The model under review builds one solid part; all positions refer to its coordinate system, in mm. A direction names the side the tool comes from. Give positions to 0.01 mm unless a question says otherwise; leave off trailing zeros. Loops run counter-clockwise (first coordinate to the right, second up) from the corner with the lowest first, then second, coordinate; pieces in that order, holes last. Notation, with made-up numbers: M -34.75,-1.75 L -22.75,-1.75 A10 cw -22.75,13.25 Z; hole C 52.5,46 d5. An arc over 180 degrees is marked long. Return JSON: item names as keys, results as strings.
Autodesk Inventor part; units mm, degrees
ref_plane "YZ Plane" through (0, 0, 0) normal (1, 0, 0) x (0, 1, 0)
ref_plane "XZ Plane" through (0, 0, 0) normal (0, 1, 0) x (-1, 0, 0)
ref_plane "XY Plane" through (0, 0, 0) normal (0, 0, 1) x (1, 0, 0)
sketch "Boceto1" plane through (0, 0, 0) normal (1, 0, 0) x (0, 1, 0)
  line L0 (0, 8) -> (10, 8)
  line L1 (10, 8) -> (10, 20)
  line L2 (10, 20) -> (0, 20)
  line L3 (20, 60) -> (0, 40)
  line L4 (0, 0) -> (20, 0)
  line L5 (40, 20) -> (20, 0)
  line L6 (20, 60) -> (40, 60)
  line L7 (0, 20) -> (0, 40)
  line L8 (0, 8) -> (0, 0)
  line L9 (40, 60) -> (120, 60)
  line L10 (120, 60) -> (120, 20)
  line L11 (80, 20) -> (80, 0)
  line L12 (80, 0) -> (120, 0)
  line L13 (120, 0) -> (120, 20)
  line L14 (40, 20) -> (80, 20)
  line L15 (120, 60) -> (115, 60)
  line L16 (120, 55) -> (120, 60)
  line L17 (20, 60) -> (25, 60)
  line L18 (120, 0) -> (115, 0)
  line L19 (120, 5) -> (120, 0)
  line L20 (0, 35) -> (0, 40)
  line L21 (0, 0) -> (5, 0)
  line L22 (0, 5) -> (0, 0)
  circle A0 centre (115, 55) radius 1.5
  circle A1 centre (115, 5) radius 1.5
  circle A2 centre (25, 55) radius 1.5
  circle A3 centre (5, 35) radius 1.5
  circle A4 centre (5, 5) radius 1.5
  line L23 (80, 0) -> (85, 0)
  line L24 (80, 5) -> (80, 0)
  circle A5 centre (85, 5) radius 1.5
  dimension "d2" = 8
  dimension "d3" = 10
  dimension "d4" = 12
  dimension "d5" = 40
  dimension "d7" = 20
  dimension "d11" = 20
  dimension "d12" = 20
  dimension "d13" = 20
  dimension "d16" = 100
  dimension "d17" = 60
  dimension "d18" = 40
  dimension "d27" = 3
  dimension "d28" = 3
  dimension "d29" = 3
  dimension "d30" = 3
  dimension "d31" = 3
  dimension "d34" = 3
  dimension "d35" = 5
  dimension "d36" = 5
  dimension "d37" = 5
  dimension "d38" = 5
  dimension "d39" = 5
  dimension "d40" = 5
  dimension "d41" = 5
  dimension "d42" = 5
  dimension "d43" = 5
  dimension "d44" = 5
  dimension "d45" = 5
  dimension "d46" = 5
extrude "Extrusión1" add sketch "Boceto1" along normal blind 5
sketch "Boceto2" plane through (5, 0, 0) normal (1, 0, 0) x (0, 0, -1)
  point P0 (0, 0)
sketch "Boceto3" plane through (5, 0, 0) normal (1, 0, 0) x (0, 0, -1)
  circle A0 centre (-25, 45) radius 1.5
  line L0 (-20, 40) -> (-20, 80)
  circle A1 centre (-45, 45) radius 1.5
  point P0 (0, 0)
  dimension "d49" = 3
  dimension "d50" = 5
  dimension "d51" = 5
  dimension "d52" = 3
  dimension "d53" = 20
  dimension "d54" = 5
extrude "Extrusión2" cut sketch "Boceto3" against normal blind 5
sketch "Boceto4" plane through (0, 0, 20) normal (0, -1, 0) x (1, 0, 0)
  point P0 (0, -20)
sketch "Boceto5" plane through (0, 0, 0) normal (0, -1, 0) x (1, 0, 0)
  circle A0 centre (2.5, 2.5) radius 1.5
  line L0 (0, 0) -> (5, 0)
  line L1 (0, 8) -> (0, 0)
  dimension "d57" = 3
  dimension "d58" = 2.5
  dimension "d59" = 2.5
extrude "Extrusión3" cut sketch "Boceto5" against normal blind 3
sketch "Boceto6" plane through (5, 0, 0) normal (1, 0, 0) x (0, 0, -1)
  line L0 (-8, 0) -> (0, 0)
  line L1 (-20.5, 10.5) -> (-7.5, 10.5)
  line L2 (-7.5, 10.5) -> (-7.5, 0)
  line L3 (-7.5, 0) -> (-20.5, 0)
  line L4 (-20.5, 0) -> (-20.5, 10.5)
  line L5 (-8, 10) -> (-8, 0)
  line L6 (-20, 0) -> (-20, 10)
  line L7 (-20, 10) -> (-8, 10)
  point P0 (-20.5, 5.25)
  dimension "d62" = 0.5
  dimension "d63" = 0.5
  dimension "d64" = 0.5
extrude "Extrusión4" cut sketch "Boceto6" against normal blind 10
sketch "Boceto7" plane through (5, 0, 0) normal (1, 0, 0) x (0, 0, -1)
  point P0 (0, 0)
sketch "Boceto8" plane through (0, 0, 40) normal (0, -1, 0) x (1, 0, 0)
  line L0 (5, -3.5) -> (0, -3.5)
  circle A0 centre (2.5, -3.5) radius 1.5
  point P0 (0, -40)
  dimension "d67" = 3
extrude "Extrusión5" cut sketch "Boceto8" against normal blind 3
sketch "Boceto9" plane through (5, 0, 0) normal (1, 0, 0) x (0, 0, -1)
  circle A0 centre (-35, 5) radius 1.5
  circle A1 centre (-35, 5) radius 1.5
  circle A2 centre (-5, 5) radius 1.5
  circle A3 centre (-5, 5) radius 1.5
  point P0 (0, 0)
extrude "Extrusión6" add sketch "Boceto9" against normal blind 5
properties part number "Lateral"
1) The part is to be moulded in two halves that separate along X. For faces 5 (the face through (0, 59, 37)), 6 (the face through (2, 3, 3)), 7 (the face through (2.46, 23.5, 54.93)), 8 (the face through (5, 59, 37)), say which applies: released by +X, released by -X, zero draft, split by the parting line, or undercut.
From the geometry:
{"face 5": "released by -X", "face 6": "undercut", "face 7": "zero draft", "face 8": "released by +X"}
2) Consider section A-A on y = 25. Write out the cut boundary in (x, z).
From the geometry:
{"outline": "M 0,5 L 5,5 L 5,53.5 L 0,53.5 Z; M 0,56.5 L 5,56.5 L 5,60 L 0,60 Z"}
3) Wall thickness on L1, parallel to Y at x = 3.75, z = 25; L2, parallel to Y at x = 4.8, z = 56; L3, parallel to Y at x = 2.25, z = 45: over which ranges is each line inside the solid? List them lowest first. Write a range as from..to.
From the geometry:
{"L1": "0..43.5, 46.5..120", "L2": "16..23.88, 26.12..113.88, 116.12..120", "L3": "5..43.5, 46.5..120"}
4) Insertion check: pin 1 (1 mm diameter, centred on x = 3, z = 23, fed in from -Y); pin 2 (1.8 mm diameter, centred on y = 45, z = 45, fed in from -X); pin 3 (1.5 mm diameter, centred on x = 3.5, y = 6, fed in from +Z); pin 4 (1.5 mm diameter, centred on x = 2.5, y = 54, fed in from -Z). Each pin has a flat end and moves straight along its axis. Give the tip position at first contact, or say it passes through.
From the geometry:
{"pin 1": "y = 0", "pin 2": "through", "pin 3": "z = 46.75", "pin 4": "z = 20"}
5) Tool access review of faces 1 (the face through (2.5, 44.1, 46.2)), 2 (the face through (2.175, 1.479, 35.036)), 3 (the face through (2, 80, 10)), 4 (the face through (3, 5, 7.5)): name each direction out of +Z, -Z, +X, -X, +Y, -Y from which nothing blocks a thin tool from reaching the whole face with its end or side.
From the geometry:
{"face 1": "+X, -X", "face 2": "-Y", "face 3": "-Z, +X, -X", "face 4": "+X, -X, -Y"}
6) Consider section C-C on z = 25. Write out the cut boundary in (x, y).
From the geometry:
{"outline": "M 0,0 L 5,0 L 5,43.5 L 0,43.5 Z; M 0,46.5 L 5,46.5 L 5,120 L 0,120 Z"}
7) Consider section D-D on y = 45. Write out the cut boundary in (x, z), then the cut area to 3 significant figures.
From the geometry:
{"outline": "M 0,20 L 5,20 L 5,23.5 L 0,23.5 Z; M 0,26.5 L 5,26.5 L 5,43.5 L 0,43.5 Z; M 0,46.5 L 5,46.5 L 5,60 L 0,60 Z", "area": "170 mm²"}
8) Consider section B-B on z = 55. Write out the cut boundary in (x, y).
From the geometry:
{"outline": "M 0,15 L 5,15 L 5,23.5 L 0,23.5 Z; M 0,26.5 L 5,26.5 L 5,113.5 L 0,113.5 Z; M 0,116.5 L 5,116.5 L 5,120 L 0,120 Z"}
